from build123d import *

# Parameters (mm, degrees)
SKETCH_1_W          = 9.58
SKETCH_1_H          = 12.27
EXTRUDE_1_DEPTH     = 6.52
SKETCH_2_W          = 7.9
SKETCH_2_H          = 1.6
CUT_EXTRUDE_1_DEPTH = 4
SKETCH_3_W          = 0.7
SKETCH_3_H          = 5.068026785
CUT_EXTRUDE_2_DEPTH = 2.5
SKETCH_4_W          = 6
SKETCH_4_H          = 4
EXTRUDE_2_DEPTH     = 1
SKETCH_5_W          = 1.79
SKETCH_5_H          = 3.771756959
CUT_EXTRUDE_3_DEPTH = 1.5
EXTRUDE_3_DEPTH     = 3
EXTRUDE_4_DEPTH     = 1.6
FILLET_1_R          = 10
SKETCH_8_W          = 7.58
SKETCH_8_H          = 4.52
CUT_EXTRUDE_4_DEPTH = 6


with BuildPart() as part:
    # 草图1 → 凸台-拉伸1 (new body)
    with BuildSketch(Plane.XY):
        with Locations((4.79, 6.135)):
            Rectangle(SKETCH_1_W, SKETCH_1_H)
    extrude(amount=EXTRUDE_1_DEPTH)

    # 草图2 → 切除-拉伸1 (cut)
    with BuildSketch(Plane.XY.offset(6.52)):
        with Locations((4.79, 7.01)):
            Rectangle(SKETCH_2_W, SKETCH_2_H)
    extrude(amount=-CUT_EXTRUDE_1_DEPTH, mode=Mode.SUBTRACT)

    # 草图3 → 切除-拉伸2 (cut)
    with BuildSketch(Plane.XY.offset(6.52)):
        with Locations((8.23, 10.008542357)):
            Rectangle(SKETCH_3_W, SKETCH_3_H)
        with Locations((6.87, 10.008542357)):
            Rectangle(SKETCH_3_W, SKETCH_3_H)
        with Locations((5.51, 10.008542357)):
            Rectangle(SKETCH_3_W, SKETCH_3_H)
        with Locations((4.15, 10.008542357)):
            Rectangle(SKETCH_3_W, SKETCH_3_H)
        with Locations((2.79, 10.008542357)):
            Rectangle(SKETCH_3_W, SKETCH_3_H)
        with Locations((1.43, 10.008542357)):
            Rectangle(SKETCH_3_W, SKETCH_3_H)
    extrude(amount=-CUT_EXTRUDE_2_DEPTH, mode=Mode.SUBTRACT)

    # 草图4 → 凸台-拉伸2 (add)
    with BuildSketch(Plane(origin=(0, 12.27, 0), x_dir=(1, 0, 0), z_dir=(0, 1, 0))):
        with Locations((4.79, -0.52)):
            Rectangle(SKETCH_4_W, SKETCH_4_H)
    extrude(amount=EXTRUDE_2_DEPTH)

    # 草图5 → 切除-拉伸3 (cut)
    with BuildSketch(Plane(origin=(0, 12.27, 0), x_dir=(1, 0, 0), z_dir=(0, 1, 0))):
        with Locations((8.685, -1.374121521)):
            Rectangle(SKETCH_5_W, SKETCH_5_H)
        with Locations((0.895, -1.374121521)):
            Rectangle(SKETCH_5_W, SKETCH_5_H)
    extrude(amount=-CUT_EXTRUDE_3_DEPTH, mode=Mode.SUBTRACT)

    # 草图6 → 凸台-拉伸3 (add, symmetric)
    with BuildSketch(Plane.ZY.offset(-4.79)):
        Polygon((-1.48, 12.27), (-1.75, 8.942581669), (-1.278125841, 8.904291917), (-1.005018858, 12.27), align=None)
    extrude(amount=EXTRUDE_3_DEPTH, both=True)

    # 草图7 → 凸台-拉伸4 (add, symmetric)
    with BuildSketch(Plane.ZY.offset(-4.79)):
        Polygon((-1.75, 8.942581669), (-4, -1.173649155), (-3.542253598, -1.275458754), (-1.278125841, 8.904291917), align=None)
    extrude(amount=EXTRUDE_4_DEPTH, both=True)

    # 圆角1
    # the kernel refuses this fillet: 10 mm, written as the material it adds along each edge
    with BuildSketch(Plane(origin=(1.79, 12.27, -1.48), x_dir=(0, -0.9967239953538545, -0.08087816198362402), z_dir=(1, 0, 0))) as fillet_1_piece_1:
        with BuildLine():
            CenterArc((FILLET_1_R * 0.0405054289786, FILLET_1_R), FILLET_1_R, 265.360955713, 4.639044287)
            Line((-FILLET_1_R * 0.040372733005, FILLET_1_R * 0.00327600464615), (0, 0))
            Line((0, 0), (FILLET_1_R * 0.0405054289786, 0))
        make_face()
    extrude(amount=6)

    # 草图8 → 切除-拉伸4 (cut)
    with BuildSketch(Plane.XZ):
        with Locations((4.79, 3.26)):
            Rectangle(SKETCH_8_W, SKETCH_8_H)
    extrude(amount=-CUT_EXTRUDE_4_DEPTH, mode=Mode.SUBTRACT)


solid = part.part
Verification items for the finished model (mm, model axes). A direction names the side the tool comes from. Round coordinates to 2 decimals unless told otherwise and drop trailing zeros. Loops run counter-clockwise (first coordinate to the right, second up) from the corner with the lowest first, then second, coordinate; pieces in that order, holes last. Notation, with made-up numbers: (62, 44.25) - (76, 44.25) arc R19 ccw to (76, 69.25) - close; hole circle Ø1 at (40, 83.25). An arc over 180 degrees is marked (long way). Answer in a Markdown table with one row per item. Add a question column.
Q1. Section check B-B on z = 2.75. Enter the section's corners in (x, y).
Q2. Material ranges on line 1 (Z direction, x = 2.5, y = 3.75); line 2 (Y direction, x = 4.75, z = 5); line 3 (X direction, y = 2.75, z = 3.5), recorded low to high.
Q3. Gauge pin test, flat ends, axial feed: pin 1 (4 mm diameter, centred on x = 7, y = 7, fed in from -Z); pin 2 (2 mm diameter, centred on x = 3, z = 4, fed in from +Y); pin 3 (1 mm diameter, centred on x = 6.5, y = 1.5, fed in from -Z). Record the tip position at first contact, or that the pin passes through.
Q4. Section check A-A on y = 5.5. Enter the section's corners in (x, z), plus the area to 3 significant figures.
Q5. Tool access check on faces 5 (the face through (9, 10.77, 2)), 6 (the face through (5, 7.81, 4)), 7 (the face through (1.78, 10, 5)), 8 (the face through (4.748, 10.564, -1.143)). Record the directions out of +Z, -Z, +X, -X, +Y, -Y that give a thin tool (end or side, any length) a straight path to the whole face; none if there is none.
Q6. Release check for a two-part mould opening along X. For faces 1 (the face through (9.58, 6, 3)), 2 (the face through (0.84, 7, 5)), 3 (the face through (5, 6, 3)), 4 (the face through (9, 12, 3.26)) record: pulls with the +X half, pulls with the -X half, needs draft (parallel to the pull), parting line crosses it, or undercut.
Q7. Section check C-C on x = 8.25. Enter the section's corners in (y, z), plus the area to 3 significant figures.
Found:
| question | item | result |
|---|---|---|
| 1 | outline | (0, 0) - (1, 0) - (1, 6) - (8.58, 6) - (8.58, 0) - (9.58, 0) - (9.58, 10.77) - (7.79, 10.77) - (7.79, 12.27) - (1.79, 12.27) - (1.79, 10.77) - (0, 10.77) - close; hole (0.84, 6.21) - (8.74, 6.21) - (8.74, 7.81) - (0.84, 7.81) - close |
| 2 | line 1 | z = 0 to 1, 5.52 to 6.52 |
| 2 | line 2 | y = 6 to 6.21, 7.81 to 12.27 |
| 2 | line 3 | x = 0 to 1, 8.58 to 9.58 |
| 3 | pin 1 | stops at z = -2.61 |
| 3 | pin 2 | stops at y = 12.27 |
| 3 | pin 3 | stops at z = -3.51 |
| 4 | outline | (0, 0) - (9.58, 0) - (9.58, 6.52) - (0, 6.52) - close; (3.19, -2.52) - (6.39, -2.52) - (6.39, -2.04) - (3.19, -2.04) - close; hole (1, 1) - (8.58, 1) - (8.58, 5.52) - (1, 5.52) - close |
| 4 | area | 29.7 mm² |
| 5 | face 5 | -Z, +X, +Y |
| 5 | face 6 | +Z |
| 5 | face 7 | +Z, +Y |
| 5 | face 8 | +X, -X, -Y |
| 6 | face 1 | pulls with the +X half |
| 6 | face 2 | undercut |
| 6 | face 3 | undercut |
| 6 | face 4 | needs draft |
| 7 | outline | (0, 0) - (10.77, 0) - (10.77, 3.26) - (12.27, 3.26) - (12.27, 4.02) - (7.81, 4.02) - (7.81, 2.52) - (6.21, 2.52) - (6.21, 6.52) - (0, 6.52) - (0, 5.52) - (6, 5.52) - (6, 1) - (0, 1) - close |
| 7 | area | 30.4 mm² |
